The drawing under review shows one solid part. Ordinate dimensions are in mm from its lowest x, y, z. A direction names the side the tool comes from. Coordinates: 2 decimals unless noted, no trailing zeros. Write each loop counter-clockwise with the first axis right and the second up, starting at its lowest first coordinate (ties: lowest second). Pieces come first, ordered by that corner, then holes. Notation, with made-up numbers: (-21.75, -0.5) - (-10.75, -0.5) arc R20 cw to (-10.75, 12.5) - close; hole circle Ø5 at (63, -8.75). An arc over 180 degrees is marked (long way). Use a Markdown table: item, result.
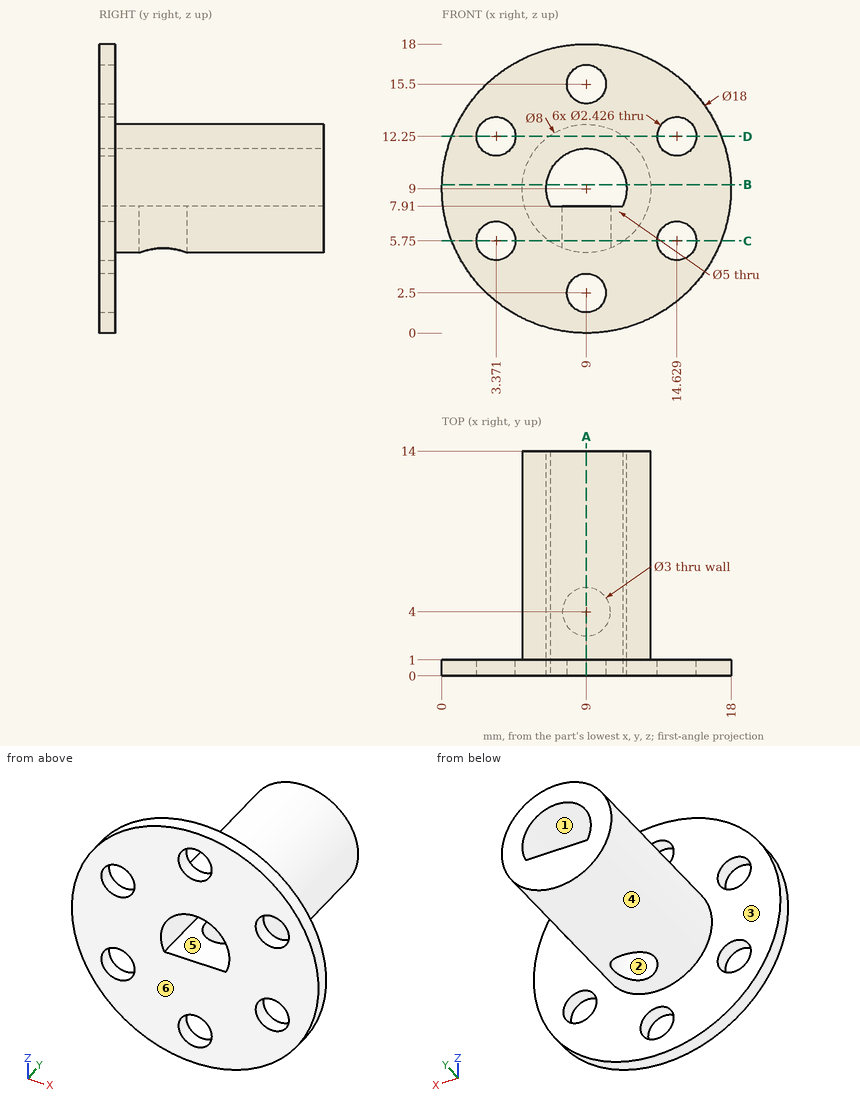
(1) For pin 1 (5 mm diameter, centred on x = 8.5, y = 5.5, fed in from +Z); pin 2 (1.9 mm diameter, centred on x = 9, z = 15.5, fed in from +Y); pin 3 (6 mm diameter, centred on y = 3.5, z = 15, fed in from -X) (1 decimal); pin 4 (4 mm diameter, centred on x = 9, y = 4, fed in from -Z), all flat-tipped, find the tip position at first contact; note any pin that passes through.
Determined:
| item | result |
|---|---|
| pin 1 | z = 13 |
| pin 2 | through |
| pin 3 | x = 1.1 |
| pin 4 | z = 5 |
(2) Machinability: for the marked faces 1, 2 and 3, which of the approach directions +Z, -Z, +X, -X, +Y, -Y give a long, thin tool a straight path to every point of the face, cutting with its end or side? Answer none if there is none.
Determined:
| item | result |
|---|---|
| face 1 | +Y, -Y |
| face 2 | -Z |
| face 3 | +Y |
(3) Take a section at D-D on z = 12.25. Write out the cut boundary in (x, y).
Determined:
| item | result |
|---|---|
| outline | (0.61, 0) - (2.16, 0) - (2.16, 1) - (0.61, 1) - close; (4.58, 0) - (13.42, 0) - (13.42, 1) - (11.33, 1) - (11.33, 14) - (6.67, 14) - (6.67, 1) - (4.58, 1) - close; (15.84, 0) - (17.39, 0) - (17.39, 1) - (15.84, 1) - close |
(4) Take a section at A-A on x = 9. Write out the cut boundary in (y, z).
Determined:
| item | result |
|---|---|
| outline | (0, 0) - (1, 0) - (1, 1.29) - (0, 1.29) - close; (0, 3.71) - (1, 3.71) - (1, 5) - (2.5, 5) - (2.5, 7.91) - (0, 7.91) - close; (0, 11.5) - (14, 11.5) - (14, 13) - (1, 13) - (1, 14.29) - (0, 14.29) - close; (0, 16.71) - (1, 16.71) - (1, 18) - (0, 18) - close; (5.5, 5) - (14, 5) - (14, 7.91) - (5.5, 7.91) - close |
(5) Draft analysis for pull direction Z (two halves, no side actions). For the marked faces 4, 5 and 6, state which applies: +Z half, -Z half, draft (parallel to the pull), parting line (faces both ways), or undercut.
Determined:
| item | result |
|---|---|
| face 4 | parting line |
| face 5 | undercut |
| face 6 | draft |
(6) Take a section at C-C on z = 5.75. Write out the cut boundary in (x, y).
Determined:
| item | result |
|---|---|
| outline | (0.61, 0) - (2.16, 0) - (2.16, 1) - (0.61, 1) - close; (4.58, 0) - (13.42, 0) - (13.42, 1) - (11.33, 1) - (11.33, 14) - (6.67, 14) - (6.67, 1) - (4.58, 1) - close; (15.84, 0) - (17.39, 0) - (17.39, 1) - (15.84, 1) - close; hole circle Ø3 at (9, 4) |
(7) Take a section at B-B on z = 9.25. Write out the cut boundary in (x, y).
Determined:
| item | result |
|---|---|
| outline | (0, 0) - (6.51, 0) - (6.51, 14) - (5.01, 14) - (5.01, 1) - (0, 1) - close; (11.49, 0) - (18, 0) - (18, 1) - (12.99, 1) - (12.99, 14) - (11.49, 14) - close |
(8) For L1, parallel to Z at x = 9, y = 0.7; L2, parallel to Z at x = 10.75, y = 12.5 (1 decimal); L3, parallel to Z at x = 7, y = 7.5 (1 decimal), list the stretches that pass through material, from the lowest coordinate up. Write a range as from..to.
Determined:
| item | result |
|---|---|
| L1 | 0..1.29, 3.71..7.91, 11.5..14.29, 16.71..18 |
| L2 | 5.4..7.9, 10.8..12.6 |
| L3 | 5.5..7.9, 10.5..12.5 |
